The figure shows three views and two pictorial views of one solid part (mm, origin at its lowest corner). Answer the questions. A direction names the side the tool comes from. Round coordinates to 2 decimals unless told otherwise and drop trailing zeros. Write each loop counter-clockwise with the first axis right and the second up, starting at its lowest first coordinate (ties: lowest second). Pieces come first, ordered by that corner, then holes. Notation, with made-up numbers: (47, 39.25) - (70, 39.25) arc R31 ccw to (70, 71.25) - close; hole circle Ø9 at (-28, -16). An arc over 180 degrees is marked (long way). Answer as CSV lines item,"result". Start each with the question number.
Item 1: Which of the six approach directions +Z, -Z, +X, -X, +Y, -Y give full straight-line access (tool end or side, diameter ignored) to the marked faces 5, 6 and 7?
Item 2: A cutting plane is placed at C-C on x = 113. Determine the outline of the cut face in (y, z) (1 decimal), and give its area (3 significant figures).
Item 3: Flat-ended cylindrical pins translate along their axes: pin 1 (6 mm diameter, centred on x = 175, y = 15.5, fed in from +Z); pin 2 (12.5 mm diameter, centred on x = 190, y = 9, fed in from -Z) (1 decimal); pin 3 (1.5 mm diameter, centred on y = 21.5, z = 100.5, fed in from +X). Find the tip coordinate at first contact, or state that the pin passes through.
Item 4: For a pull along X with two mould halves and no side action, classify the marked faces 1, 2, 3 and 4 as pulls with the +X half, pulls with the -X half, needs draft (parallel to the pull), parting line crosses it, or undercut.
Item 5: A cutting plane is placed at D-D on z = 106.5. Determine the outline of the cut face in (x, y) (1 decimal).
Item 6: Straight lines are drawn through the part: line 1 along X through (y, z) = (4.75, 58); line 2 along Z through (x, y) = (127, 4.75) (1 decimal); line 3 along X through (y, z) = (9, 77) (1 decimal). For each, find the intervals that lie inside material, in ascending order. Write a range as [from, to].
Item 7: A cutting plane is placed at A-A on z = 60. Determine the outline of the cut face in (x, y), and give its area (3 significant figures).
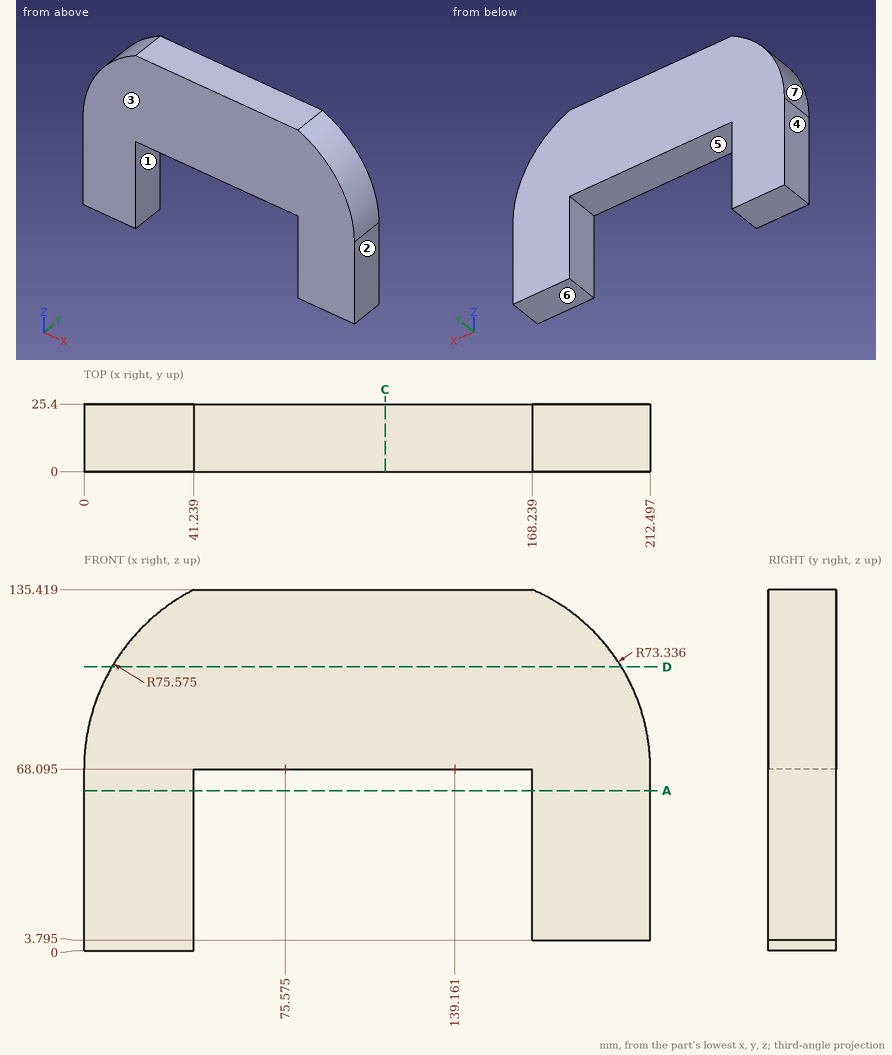
Geometry says:
1,face 5,"-Z, +Y, -Y"
1,face 6,"-Z, +X, +Y, -Y"
1,face 7,"+Z, -X, +Y, -Y"
2,outline,"(0, 68.1) - (25.4, 68.1) - (25.4, 135.4) - (0, 135.4) - close"
2,area,"1,710 mm^2"
3,pin 1,"stops at z = 133.67"
3,pin 2,"stops at z = 3.8"
3,pin 3,"stops at x = 205.31"
4,face 1,"undercut"
4,face 2,"pulls with the +X half"
4,face 3,"needs draft"
4,face 4,"pulls with the -X half"
5,outline,"(10.5, 0) - (201.6, 0) - (201.6, 25.4) - (10.5, 25.4) - close"
6,line 1,"x = [0, 41.24], [168.24, 212.5]"
6,line 2,"z = [68.1, 135.4]"
6,line 3,"x = [0.5, 212]"
7,outline,"(0, 0) - (41.24, 0) - (41.24, 25.4) - (0, 25.4) - close; (168.24, 0) - (212.5, 0) - (212.5, 25.4) - (168.24, 25.4) - close"
7,area,"2,170 mm^2"
